```python
from build123d import *

# Parameters (mm, degrees)
SKETCH_1_R               = 10
SKETCH_1_R_2             = 3.1
EXTRUDE_1_DEPTH          = 15
SKETCH_2_R               = 32
EXTRUDE_2_DEPTH          = 5
SKETCH_3_R               = 7.5
EXTRUDE_3_DEPTH          = 10
SKETCH_4_R               = 17.5
EXTRUDE_4_DEPTH          = 5
SKETCH_5_R               = 1.85
CUT_EXTRUDE_1_DEPTH      = 33
SKETCH_5_3_R             = 1.25
CUT_EXTRUDE_2_DEPTH      = 33
CUT_EXTRUDE_2_DEPTH_BACK = 33
FILLET_1_R               = 4


with BuildPart() as part:
    # Sketch 1 → Extrude 1 (new body)
    with BuildSketch(Plane.XY):
        Circle(SKETCH_1_R)
        Circle(SKETCH_1_R_2, mode=Mode.SUBTRACT)
    extrude(amount=EXTRUDE_1_DEPTH)

    # Sketch 2 → Extrude 2 (add)
    with BuildSketch(Plane.XY):
        Circle(SKETCH_2_R)
    extrude(amount=-EXTRUDE_2_DEPTH)

    # Sketch 3 → Extrude 3 (add)
    with BuildSketch(Plane(origin=(0, 0, -5), x_dir=(-1, 0, 0), z_dir=(0, 0, -1))):
        Circle(SKETCH_3_R)
    extrude(amount=EXTRUDE_3_DEPTH)

    # Sketch 4 → Extrude 4 (add)
    with BuildSketch(Plane(origin=(0, 0, -15), x_dir=(-1, 0, 0), z_dir=(0, 0, -1))):
        Circle(SKETCH_4_R)
    extrude(amount=EXTRUDE_4_DEPTH)

    # Sketch 5 → Cut-Extrude 1 (cut, through all)
    with BuildSketch(Plane(origin=(0, 0, 0), x_dir=(1, 0, 0), z_dir=(0, 1, 0))):
        with Locations((0, -8.5)):
            Circle(SKETCH_5_R)
    extrude(amount=-CUT_EXTRUDE_1_DEPTH, mode=Mode.SUBTRACT)

    # Sketch 5_3 → Cut-Extrude 2 (cut, two sides)
    with BuildSketch(Plane(origin=(0, 0, 0), x_dir=(1, 0, 0), z_dir=(0, 1, 0))) as cut_extrude_2_sk:
        with Locations((0, 10)):
            Circle(SKETCH_5_3_R)
    extrude(amount=CUT_EXTRUDE_2_DEPTH, mode=Mode.SUBTRACT)
    extrude(cut_extrude_2_sk.sketch, amount=-CUT_EXTRUDE_2_DEPTH_BACK, mode=Mode.SUBTRACT)

    # Fillet 1
    fillet_1_edges = [part.edges().sort_by_distance(p)[0] for p in [
        (-32, 0, -5),
        (7.5, 0, -5),
        (7.5, 0, -15),
        (17.5, 0, -15),
    ]]
    fillet(fillet_1_edges, radius=FILLET_1_R)


solid = part.part
```
Source: CAD feature listing. Evaluate the final solid. Frame: model axes, mm. A direction names the side the tool comes from. Round coordinates to 2 decimals unless told otherwise and drop trailing zeros. Loops run counter-clockwise (first coordinate to the right, second up) from the corner with the lowest first, then second, coordinate; pieces in that order, holes last. Notation, with made-up numbers: M 52.5,-13 L 67.5,-13 A25 cw 67.5,25 Z; hole C -7,-38.5 d8. An arc over 180 degrees is marked long. Use a Markdown table: item, result. Add a question column.
1. Contact query for flat-ended pins moving along their axis: pin 1 (6 mm diameter, centred on y = -22.5, z = -1, fed in from -X); pin 2 (12 mm diameter, centred on x = -6, z = -12.5, fed in from -Y); pin 3 (12 mm diameter, centred on x = -16.5, z = -8, fed in from +Y); pin 4 (7 mm diameter, centred on x = -1, y = 1.5, fed in from +Z). Output: stop coordinate, or through.
2. Cut plane D-D, the plane z = -16. Output: boundary loops of the cut face in (x, y), and give its area (3 significant figures).
3. Set-up query: faces 1 (the flat face through (0, 0, 0)), 2 (the cylindrical face through (-7.5, -0.15, -9.99)), 3 (the cylindrical face through (13.887, -10.648, -19.493)), 4 (the flat face through (-10, 6, -15)). Return all of +Z, -Z, +X, -X, +Y, -Y with unobstructed straight access to the full face (end or side cutting, diameter ignored); none if empty.
4. Pull-direction query (X, two-part tool) for faces 5 (the cylindrical face through (7.5, 0.15, -9.99)), 6 (the cylindrical face through (-2.17, -9.76, 7.4)), 7 (the cylindrical face through (-0.404, 3.074, 7.395)), 8 (the flat face through (0, -12, -5)); classes: +X half, -X half, draft (parallel to the pull), parting line (faces both ways), or undercut.
5. Ray query, line 1 along Z through (x, y) = (0, -4.25); line 2 along Y through (x, z) = (0, 6.5); line 3 along Z through (x, y) = (0, 1). Return the intervals inside material, ascending. Write a range as [from, to].
6. Cut plane C-C, the plane z = 8.5. Output: boundary loops of the cut face in (x, y).
7. Cut plane B-B, the plane z = -10. Output: boundary loops of the cut face in (x, y), and give its area (3 significant figures).
Solution:
| question | item | result |
|---|---|---|
| 1 | pin 1 | stops at x = -25.37 |
| 1 | pin 2 | stops at y = -17.02 |
| 1 | pin 3 | stops at y = 28.57 |
| 1 | pin 4 | stops at z = 15 |
| 2 | outline | C 0,0 d32.29 |
| 2 | area | 819 mm2 |
| 3 | face 1 | +Z |
| 3 | face 2 | -X |
| 3 | face 3 | -Z |
| 3 | face 4 | none |
| 4 | face 5 | +X half |
| 4 | face 6 | parting line |
| 4 | face 7 | undercut |
| 4 | face 8 | draft |
| 5 | line 1 | z = [-20, -11.25], [-8.75, 6.65], [10.35, 15] |
| 5 | line 2 | y = [-10, -3.1], [3.1, 10] |
| 5 | line 3 | z = [-20, -11.25], [-8.75, 0] |
| 6 | outline | M -1.85,-9.83 L -1.85,-2.49 A3.1 cw long 1.85,-2.49 L 1.85,-9.83 A10 ccw long Z |
| 7 | outline | M -1.25,-7.4 L -1.25,7.4 A7.5 ccw Z; M 1.25,-7.4 A7.5 ccw 1.25,7.4 Z |
| 7 | area | 139 mm2 |
